Work out the finished part from the listing and answer in its coordinate system (mm). A direction names the side the tool comes from. Round coordinates to 2 decimals unless told otherwise and drop trailing zeros. Loops run counter-clockwise (first coordinate to the right, second up) from the corner with the lowest first, then second, coordinate; pieces in that order, holes last. Notation, with made-up numbers: M 45.25,51.25 L 87.25,51.25 A36 ccw 87.25,86.25 Z; hole C -17,26.5 d9. An arc over 180 degrees is marked long. One line per item, written item: value.
```python
from build123d import *

# Parameters (mm, degrees)
SKETCH1_R                    = 15.5
SKETCH1_R_2                  = 7.8
BOSS_EXTRUDE1_DEPTH          = 24
SKETCH2_R                    = 2.5
SKETCH2_R_2                  = 7.8
BOSS_EXTRUDE2_DEPTH          = 5
SKETCH4_R                    = 2.5
SKETCH4_R_2                  = 7.8
BOSS_EXTRUDE3_DEPTH          = 3
BOSS_EXTRUDE4_DEPTH          = 15
CHAMFER1_SIZE                = 3
CHAMFER2_SIZE                = 2
CHAMFER3_SIZE                = 5
CUT_EXTRUDE_THIN1_DEPTH      = 51.568623258
CUT_EXTRUDE_THIN1_DEPTH_BACK = 50
SKETCH6_W                    = 28.833380518
SKETCH6_H                    = 1
SKETCH7_R                    = 32.954924651
CUT_EXTRUDE1_DEPTH           = 5


with BuildPart() as part:
    # Sketch1 → Boss-Extrude1 (new body)
    with BuildSketch(Plane.XY):
        Circle(SKETCH1_R)
        Circle(SKETCH1_R_2, mode=Mode.SUBTRACT)
    extrude(amount=BOSS_EXTRUDE1_DEPTH)

    # Sketch2 → Boss-Extrude2 (add)
    with BuildSketch(Plane(origin=(0, 0, 0), x_dir=(-1, 0, 0), z_dir=(0, 0, -1))):
        with BuildLine():
            Line((30, -7.5), (13.564659966, -7.5))
            ThreePointArc((13.564659966, -7.5), (-15.5, 0), (13.564659966, 7.5))
            Line((13.564659966, 7.5), (30, 7.5))
            ThreePointArc((30, 7.5), (37.5, 0), (30, -7.5))
        make_face()
        with Locations((30, 0)):
            Circle(SKETCH2_R, mode=Mode.SUBTRACT)
        with Locations(Location((0, 0, 0), (0, 0, 180))):
            Circle(SKETCH2_R_2, mode=Mode.SUBTRACT)
    extrude(amount=-BOSS_EXTRUDE2_DEPTH)



with BuildPart() as body_2:
    # Sketch4 → Boss-Extrude3 (new body)
    with BuildSketch(Plane(origin=(0, 0, -2.2), x_dir=(-1, 0, 0), z_dir=(0, 0, -1))):
        with BuildLine():
            Line((13.564659966, -7.5), (30, -7.5))
            ThreePointArc((30, -7.5), (37.5, 0), (30, 7.5))
            Line((30, 7.5), (13.564659966, 7.5))
            ThreePointArc((13.564659966, 7.5), (-15.5, 0), (13.564659966, -7.5))
        make_face()
        with Locations((30, 0)):
            Circle(SKETCH4_R, mode=Mode.SUBTRACT)
        with Locations(Location((0, 0, 0), (0, 0, 180))):
            Circle(SKETCH4_R_2, mode=Mode.SUBTRACT)
    extrude(amount=BOSS_EXTRUDE3_DEPTH)


with BuildPart() as part_1:
    add(part.part)

    add(body_2.part)  # Boss-Extrude4 merges body 2
    # Sketch5 → Boss-Extrude4 (add)
    with BuildSketch(Plane(origin=(0, 0, -5.2), x_dir=(-1, 0, 0), z_dir=(0, 0, -1))):
        with BuildLine():
            Line((-6.629807067, -17.27123789), (-5.554703218, -14.470496611))
            ThreePointArc((-5.554703218, -14.470496611), (-15.5, 0), (-5.554703218, 14.470496611))
            Line((-5.554703218, 14.470496611), (-6.629807067, 17.27123789))
            ThreePointArc((-6.629807067, 17.27123789), (-18.5, 0), (-6.629807067, -17.27123789))
        make_face()
    extrude(amount=-BOSS_EXTRUDE4_DEPTH)

    # Chamfer1
    chamfer1_edges = [part_1.edges().sort_by_distance(p)[0] for p in [
        (12.773955924, -8.779296672, 9.8),
    ]]
    chamfer(chamfer1_edges, length=CHAMFER1_SIZE - 0.0001)  # a hair under: the kernel refuses the full size

    # Chamfer2
    chamfer2_edges = [part_1.edges().sort_by_distance(p)[0] for p in [
        (18.5, 0, -5.2),
    ]]
    chamfer(chamfer2_edges, length=CHAMFER2_SIZE)

    # Chamfer3
    chamfer3_edges = [part_1.edges().sort_by_distance(p)[0] for p in [
        (-15.5, 0, 5),
    ]]
    chamfer(chamfer3_edges, length=CHAMFER3_SIZE)

    # Sketch6 → Cut-Extrude-Thin1 (cut, two sides: drawn at the far end of the back side and taken through both)
    with BuildSketch(Plane.XY.offset(24).offset(-CUT_EXTRUDE_THIN1_DEPTH_BACK)):
        with Locations((14.416690259, 0)):
            Rectangle(SKETCH6_W, SKETCH6_H)
    extrude(amount=CUT_EXTRUDE_THIN1_DEPTH + CUT_EXTRUDE_THIN1_DEPTH_BACK, mode=Mode.SUBTRACT)

    # Sketch7 → Cut-Extrude1 (cut)
    with BuildSketch(Plane(origin=(22.2, 0, 0), x_dir=(0, 0, -1), z_dir=(1, 0, 0))):
        with Locations((-8.942536343, 0)):
            Circle(SKETCH7_R)
    extrude(amount=-CUT_EXTRUDE1_DEPTH, mode=Mode.SUBTRACT)


solid = part_1.part
```
1) The mould has two halves that part along X. Classify faces 1 (the face through (12.557, -9.088, -1.115)), 2 (the face through (-11, 0, -2.2)), 3 (the face through (13.23, -9.54, 11.99)), 4 (the face through (-27.5, 0.1, -3.7)): +X half, -X half, draft (parallel to the pull), parting line (faces both ways), or undercut.
Check values:
face 1: -X half
face 2: draft
face 3: +X half
face 4: undercut
2) Each of these flat-tipped pins is pushed along its axis until it touches: pin 1 (11 mm diameter, centred on x = -23, z = 7, fed in from +Y); pin 2 (4.5 mm diameter, centred on x = -28, y = -2, fed in from +Z); pin 3 (1 mm diameter, centred on x = 3, z = 20, fed in from +Y). Where does it stop, or does it pass through?
Check values:
pin 1: y = 7.5
pin 2: z = 5
pin 3: y = 15.3
3) Find section D-D (y = 4). Give the number of separate pieces and of enclosed holes in the cut face, then the cut area to 3 significant figures.
Check values:
separate pieces: 3
enclosed holes: 0
area: 668 mm2
4) Find section B-B (z = 7.5). Give the vertices of the cut face in (x, y), then the cut area to 3 significant figures.
Check values:
outline: M -16.36,-7.5 L -13.56,-7.5 A15.5 ccw 5.55,-14.47 L 6.63,-17.27 A18.5 ccw 17.2,-6.81 L 17.2,-0.5 L 7.78,-0.5 A7.8 cw long 7.78,0.5 L 17.2,0.5 L 17.2,6.81 A18.5 ccw 6.63,17.27 L 5.55,14.47 A15.5 ccw -13.56,7.5 L -16.36,7.5 A18 ccw Z
area: 704 mm2
5) Find section A-A (x = 0). Give the vertices of the cut face in (y, z), then the cut area to 3 significant figures.
Check values:
outline: M -15.5,-5.2 L -7.8,-5.2 L -7.8,-2.2 L -15.5,-2.2 Z; M -15.5,0 L -7.8,0 L -7.8,24 L -15.5,24 Z; M 7.8,-5.2 L 15.5,-5.2 L 15.5,-2.2 L 7.8,-2.2 Z; M 7.8,0 L 15.5,0 L 15.5,24 L 7.8,24 Z
area: 416 mm2
6) For faces 5 (the face through (12.704, 8.88, -1.115)), 6 (the face through (6.1, -15.89, 3.67)), 7 (the face through (-7.793, -0.336, -3.679)), determine the directions among +Z, -Z, +X, -X, +Y, -Y from which every point of the face is accessible in a straight line to the end or side of a thin tool.
Check values:
face 5: -X
face 6: +Z, -Z, -Y
face 7: +Z, -Z
7) Find section C-C (x = -12). Give the vertices of the cut face in (y, z).
Check values:
outline: M -9.81,-5.2 L 9.81,-5.2 L 9.81,-2.2 L -9.81,-2.2 Z; M -9.81,0 L 9.81,0 L 9.81,24 L -9.81,24 Z
8) Find the intervals of material crossed by probe 1 along Y at (x, z) = (0, -3.45); probe 2 along Y at (x, z) = (-30, -4.3); probe 3 along Z at (x, y) = (11, 2.5), in increasing order. Write a range as from..to.
Check values:
probe 1: -15.5..-7.8, 7.8..15.5
probe 2: -7.5..-2.5, 2.5..7.5
probe 3: -5.2..-2.2, 0..24
